from build123d import *

# Parameters (mm, degrees)
F2_DEPTH = 177.8
F3_DEPTH = 19.05
F1_W     = 482.6
F1_H     = 50.8
F4_DEPTH = 19.05


# Not quite as in the source:
# - a feature names something its author has since deleted; it is built from what else it names


with BuildPart() as f2:
    # F0 (on Front) → F2 (new body)
    with BuildSketch(Plane.XZ):
        with BuildLine():
            Line((-254, -127), (254, -127))
            ThreePointArc((254, -127), (258.4901280605, -125.1401280605), (260.35, -120.65))
            Line((260.35, -120.65), (260.35, 120.65))
            ThreePointArc((260.35, 120.65), (258.4901280605, 125.1401280605), (254, 127))
            Line((254, 127), (-254, 127))
            ThreePointArc((-254, 127), (-258.4901280605, 125.1401280605), (-260.35, 120.65))
            Line((-260.35, 120.65), (-260.35, -120.65))
            ThreePointArc((-260.35, -120.65), (-258.4901280605, -125.1401280605), (-254, -127))
        make_face()
        Polygon((222.25, 107.95), (241.3, 107.95), (241.3, -107.95), (222.25, -107.95), (-222.25, -107.95), (-241.3, -107.95), (-241.3, 107.95), (-222.25, 107.95), align=None, mode=Mode.SUBTRACT)
    extrude(amount=-F2_DEPTH)

    # F1 (on face) → F3 (join)
    with BuildSketch(Plane.XZ):
        Polygon((-222.25, 107.95), (-241.0535812378, 107.95), (-241.0535812378, 57.6071217656), (241.3, 57.6071217656), (241.3, 107.95), (222.25, 107.95), align=None)
    extrude(amount=-F3_DEPTH)

    # F1 (on face) → F4 (join)
    with BuildSketch(Plane.XZ):
        with Locations((0.2464187622, 83.0071217656)):
            Rectangle(F1_W, F1_H)
        with BuildLine():
            Line((-102.1507469177, -49.3358883619), (-0.5507469177, -49.3358883619))
            Line((-0.5507469177, -49.3358883619), (101.0492530823, -49.3358883619))
            ThreePointArc((101.0492530823, -49.3358883619), (105.5393811428, -51.1957603014), (107.3992530823, -55.6858883619))
            Line((107.3992530823, -55.6858883619), (113.2842159033, -107.1381363198))
            Line((113.2842159033, -107.1381363198), (240.2842159033, -107.1381363198))
            Line((240.2842159033, -107.1381363198), (240.2842159033, -18.2381363198))
            Line((240.2842159033, -18.2381363198), (-242.3157840967, -18.2381363198))
            Line((-242.3157840967, -18.2381363198), (-242.3157840967, -107.1381363198))
            Line((-242.3157840967, -107.1381363198), (-115.3157840967, -107.1381363198))
            Line((-115.3157840967, -107.1381363198), (-108.5007469177, -55.6858883619))
            ThreePointArc((-108.5007469177, -55.6858883619), (-106.6408749783, -51.1957603014), (-102.1507469177, -49.3358883619))
        make_face()
    extrude(amount=-F4_DEPTH)


solid = f2.part
Can you work these out from the model? Positions are in its coordinate system, mm. A direction names the side the tool comes from. Give positions to 0.01 mm unless a question says otherwise; leave off trailing zeros. Write each loop counter-clockwise with the first axis right and the second up, starting at its lowest first coordinate (ties: lowest second). Pieces come first, ordered by that corner, then holes. Notation, with made-up numbers: (89, 7) -> (116, 7) arc R31 cw to (116, 35) -> close; hole circle Ø8 at (-13, 29.25). An arc over 180 degrees is marked (long way). Answer as a JSON object with one key per item and string values. Group by question number.
Item 1: I'm going to push a flat-ended pin straight in: P1, Ø15, axis at x = -39, z = 82.5, coming from the +Y side. Where does the tip first touch, or does it pass through?
Item 2: For faces 4 (the face through (3, 88, -107.95)), 5 (the face through (-4, 19.05, -42)), 6 (the face through (4, 88, 127)), which set-ups out of +Z, -Z, +X, -X, +Y, -Y let a thin tool reach every point of the face, with its end or its side?
Item 3: Suppose I cut it at B-B (x = -125). Please give me the cut outline in (y, z), plus the area to 3 significant figures.
Item 4: Suppose I cut it at C-C (y = 141). Please give me the cut outline in (x, z), plus the area to 3 significant figures.
Item 5: Suppose I cut it at D-D (z = -84). Please give me the cut outline in (x, y).
Item 6: Suppose I cut it at A-A (z = 44). Please give me the cut outline in (x, y), plus the area to 3 significant figures.
Item 7: We'd pull the mould along Z, two halves only. Please class faces 1 (the face through (-21, 177.8, -112)), 2 (the face through (-4, 88, -127)), 3 (the face through (110.3, 9.39, -81.05)): +Z half, -Z half, draft (parallel to the pull), parting line (faces both ways), or undercut.
Item 8: Please list where these lines run through material, in increasing order: line 1 (X direction, y = 56.5, z = -86.5); line 2 (Z direction, x = -19, y = 105); line 3 (Y direction, x = -191.5, z = -102). Write a range as [from, to].
Findings:
{
 "1": {"P1": "stops at y = 19.05"},
 "2": {"face 4": "+Y, -Y", "face 5": "+Y", "face 6": "+Z, +X, -X, +Y, -Y"},
 "3": {"outline": "(0, -127) -> (177.8, -127) -> (177.8, -107.95) -> (0, -107.95) -> close; (0, -107.14) -> (19.05, -107.14) -> (19.05, -18.24) -> (0, -18.24) -> close; (0, 57.61) -> (19.05, 57.61) -> (19.05, 107.95) -> (177.8, 107.95) -> (177.8, 127) -> (0, 127) -> close", "area": "9,430 mm²"},
 "4": {"outline": "(-260.35, -120.65) arc R6.35 ccw to (-254, -127) -> (254, -127) arc R6.35 ccw to (260.35, -120.65) -> (260.35, 120.65) arc R6.35 ccw to (254, 127) -> (-254, 127) arc R6.35 ccw to (-260.35, 120.65) -> close; hole (-241.3, -107.95) -> (241.3, -107.95) -> (241.3, 107.95) -> (-241.3, 107.95) -> close", "area": "28,000 mm²"},
 "5": {"outline": "(-260.35, 0) -> (-112.25, 0) -> (-112.25, 19.05) -> (-241.3, 19.05) -> (-241.3, 177.8) -> (-260.35, 177.8) -> close; (110.64, 0) -> (240.28, 0) -> (240.28, 19.05) -> (110.64, 19.05) -> close; (241.3, 0) -> (260.35, 0) -> (260.35, 177.8) -> (241.3, 177.8) -> close"},
 "6": {"outline": "(-260.35, 0) -> (-241.3, 0) -> (-241.3, 177.8) -> (-260.35, 177.8) -> close; (241.3, 0) -> (260.35, 0) -> (260.35, 177.8) -> (241.3, 177.8) -> close", "area": "6,770 mm²"},
 "7": {"face 1": "draft", "face 2": "-Z half", "face 3": "undercut"},
 "8": {"line 1": "x = [-260.35, -241.3], [241.3, 260.35]", "line 2": "z = [-127, -107.95], [107.95, 127]", "line 3": "y = [0, 19.05]"}
}
